from build123d import *

# Parameters (mm, degrees)
BOSS_EXTRUDE1_DEPTH     = 3
CUT_EXTRUDE1_DEPTH      = 1.0000001
CUT_EXTRUDE1_DEPTH_BACK = 3
CUT_EXTRUDE2_DEPTH      = 1.0000001
CUT_EXTRUDE2_DEPTH_BACK = 3
CUT_EXTRUDE3_DEPTH      = 1.0000001
CUT_EXTRUDE3_DEPTH_BACK = 3
CUT_EXTRUDE4_DEPTH      = 1.0000001
CUT_EXTRUDE4_DEPTH_BACK = 3


with BuildPart() as part:
    # Sketch1 → Boss-Extrude1 (new body)
    with BuildSketch(Plane.XY):
        with BuildLine():
            Line((-80, 41.231056256), (-28, 41.231056256))
            Line((-28, 41.231056256), (-27.5, 48.233227348))
            Line((-27.5, 48.233227348), (-27, 48.233227348))
            Line((-27, 48.233227348), (-27, 39.233227348))
            Line((-27, 39.233227348), (-27.5, 38.233227348))
            Line((-27.5, 38.233227348), (-28, 37.733227348))
            Line((-28, 37.733227348), (-28, 36.733227348))
            Line((-28, 36.733227348), (-26.5, 35.233227348))
            Line((-26.5, 35.233227348), (-25, 35.233227348))
            Line((-25, 35.233227348), (-24.5, 48.233227348))
            Line((-24.5, 48.233227348), (-24, 48.233227348))
            Line((-24, 48.233227348), (-24, 35.233227348))
            Line((-24, 35.233227348), (-16, 35.233227348))
            Line((-16, 35.233227348), (-16, 48.233227348))
            Line((-16, 48.233227348), (-15.5, 48.233227348))
            Line((-15.5, 48.233227348), (-15, 35.233227348))
            Line((-15, 35.233227348), (-13.5, 35.233227348))
            Line((-13.5, 35.233227348), (-12, 36.733227348))
            Line((-12, 36.733227348), (-12, 37.733227348))
            Line((-12, 37.733227348), (-12.5, 38.233227348))
            Line((-12.5, 38.233227348), (-13, 39.233227348))
            Line((-13, 39.233227348), (-13, 48.233227348))
            Line((-13, 48.233227348), (-12.5, 48.233227348))
            Line((-12.5, 48.233227348), (-12, 41.231056256))
            Line((-12, 41.231056256), (52, 41.231056256))
            Line((52, 41.231056256), (52.5, 48.233227348))
            Line((52.5, 48.233227348), (53, 48.233227348))
            Line((53, 48.233227348), (53, 39.233227348))
            Line((53, 39.233227348), (52.5, 38.233227348))
            Line((52.5, 38.233227348), (52, 37.733227348))
            Line((52, 37.733227348), (52, 36.733227348))
            Line((52, 36.733227348), (53.5, 35.233227348))
            Line((53.5, 35.233227348), (55, 35.233227348))
            Line((55, 35.233227348), (55.5, 48.233227348))
            Line((55.5, 48.233227348), (56, 48.233227348))
            Line((56, 48.233227348), (56, 35.233227348))
            Line((56, 35.233227348), (64, 35.233227348))
            Line((64, 35.233227348), (64, 48.233227348))
            Line((64, 48.233227348), (64.5, 48.233227348))
            Line((64.5, 48.233227348), (65, 35.233227348))
            Line((65, 35.233227348), (66.5, 35.233227348))
            Line((66.5, 35.233227348), (68, 36.733227348))
            Line((68, 36.733227348), (68, 37.733227348))
            Line((68, 37.733227348), (67.5, 38.233227348))
            Line((67.5, 38.233227348), (67, 39.233227348))
            Line((67, 39.233227348), (67, 48.233227348))
            Line((67, 48.233227348), (67.5, 48.233227348))
            Line((67.5, 48.233227348), (68, 41.231056256))
            Line((68, 41.231056256), (80, 41.231056256))
            add(Edge.make_bspline(
                [(80, 41.231056256), (80, 105.23), (0, 105.23)],
                knots=[0, 0, 0, 1.570796327, 1.570796327, 1.570796327], degree=2, weights=[1, 0.707106781, 1]))
            add(Edge.make_bspline(
                [(0, 105.23), (-80, 105.23), (-80, 41.231056256)],
                knots=[1.570796327, 1.570796327, 1.570796327, 3.141592654, 3.141592654, 3.141592654], degree=2, weights=[1, 0.707106781, 1]))
        make_face()
    extrude(amount=BOSS_EXTRUDE1_DEPTH)

    # Sketch8 → Cut-Extrude1 (cut, two sides)
    with BuildSketch(Plane.XY.offset(3)) as cut_extrude1_sk:
        Polygon((-68, -291.258415465), (-68, 41.231056256), (-68, 45.231056256), (-52, 45.231056256), (-52, 41.231056256), (-52, -291.258415465), (-52, -956.237358907), (-68, -956.237358907), align=None)
    extrude(amount=CUT_EXTRUDE1_DEPTH, mode=Mode.SUBTRACT)
    extrude(cut_extrude1_sk.sketch, amount=-CUT_EXTRUDE1_DEPTH_BACK, mode=Mode.SUBTRACT)

    # Sketch9 → Cut-Extrude2 (cut, two sides)
    with BuildSketch(Plane.XY.offset(3)) as cut_extrude2_sk:
        Polygon((28, -219.845544284), (28, 41.231056256), (28, 45.231056256), (12, 45.231056256), (12, 41.231056256), (12, -219.845544284), (12, -741.998745365), (28, -741.998745365), align=None)
    extrude(amount=CUT_EXTRUDE2_DEPTH, mode=Mode.SUBTRACT)
    extrude(cut_extrude2_sk.sketch, amount=-CUT_EXTRUDE2_DEPTH_BACK, mode=Mode.SUBTRACT)

    # Sketch10 → Cut-Extrude3 (cut, two sides)
    with BuildSketch(Plane.XY.offset(3)) as cut_extrude3_sk:
        Polygon((-1.500000233, 330.069612224), (-1.500000233, 105.218749193), (-1.500000233, 73.231), (1.499999767, 73.231), (1.499999767, 105.2187492), (1.499999767, 330.069612231), (1.499998719, 779.771338291), (-1.500001281, 779.771338284), align=None)
    extrude(amount=CUT_EXTRUDE3_DEPTH, mode=Mode.SUBTRACT)
    extrude(cut_extrude3_sk.sketch, amount=-CUT_EXTRUDE3_DEPTH_BACK, mode=Mode.SUBTRACT)

    # Sketch11 → Cut-Extrude4 (cut, two sides)
    with BuildSketch(Plane.XY.offset(3)) as cut_extrude4_sk:
        Polygon((-46.64838896, 381.810733149), (-46.64838896, 93.22359963), (-46.64838896, 67.904187559), (-43.64838896, 67.904187559), (-43.64838896, 94.864894992), (-43.64838896, 383.452028511), (-320.670818857, 889.800434121), (-323.670818857, 888.159138759), align=None)
    extrude(amount=CUT_EXTRUDE4_DEPTH, mode=Mode.SUBTRACT)
    extrude(cut_extrude4_sk.sketch, amount=-CUT_EXTRUDE4_DEPTH_BACK, mode=Mode.SUBTRACT)


solid = part.part
Geometry: final body of the model. Coordinates: model frame, mm. A direction names the side the tool comes from. Round coordinates to 2 decimals unless told otherwise and drop trailing zeros.
Q1. Material intervals for probe 1 along X at (y, z) = (75, 1.7); probe 2 along X at (y, z) = (94, 0.2); probe 3 along X at (y, z) = (56.5, 0.35), sorted ascending.
Result sheet:
probe 1: x = -67.96 to -46.65, -43.65 to -1.5, 1.5 to 67.96
probe 2: x = -43.65 to -1.5, 1.5 to 45.27
probe 3: x = -77.69 to 77.69
Q2. Mould query, pull axis Y, two halves, no side actions, for faces 5 (the face through (40, 41.231, 1)), 6 (the face through (-1.5, 89, 2)), 7 (the face through (67, 44, 1)). Classes: released by +Y, released by -Y, zero draft, split by the parting line, or undercut.
Result sheet:
face 5: released by -Y
face 6: zero draft
face 7: undercut
Q3. Section A-A, the plane y = 84.5. Give the number of separate pieces and of enclosed holes in the cut face, and give its area (3 significant figures).
Result sheet:
separate pieces: 3
enclosed holes: 0
area: 336 mm2
Q4. Pin query (flat end, axial travel): pin 1 (0.9 mm diameter, centred on y = 91, z = 1, fed in from +X); pin 2 (0.9 mm diameter, centred on x = -44.5, z = 1.5, fed in from +Y); pin 3 (1.1 mm diameter, centred on y = 37, z = 2, fed in from -X); pin 4 (10 mm diameter, centred on x = -57.5, y = 66, fed in from -Z). Return the tip coordinate at first contact, or that it passes through.
Result sheet:
pin 1: stops at x = 50.98
pin 2: stops at y = 67.9
pin 3: stops at x = -28
pin 4: stops at z = 0
Q5. Access query for faces 1 (the face through (-24, 42, 1)), 2 (the face through (-45, 67.904, 2)), 3 (the face through (-12.254, 44.781, 1.479)), 4 (the face through (-74, 41.231, 1)). Directions: +Z, -Z, +X, -X, +Y, -Y. A direction counts if a zero-diameter tool reaches every point of the face in a straight line with its end or side. Return the directions, or none.
Result sheet:
face 1: +Z, -Z, -Y
face 2: +Z, -Z, +Y
face 3: +Z, -Z
face 4: +Z, -Z, -X, -Y
